```python
from build123d import *

# Parameters (mm, degrees)
F0_W     = 55
F0_H     = 55
F1_DEPTH = 20
F3_W     = 28
F3_H     = 28
F4_DEPTH = 13
F5_W     = 55
F5_H     = 55
F5_W_2   = 43
F5_H_2   = 43
F6_DEPTH = 9
F8_DEPTH = 22.5


with BuildPart() as f1:
    # F0 (on Top) → F1 (new body)
    with BuildSketch(Plane.XY):
        Rectangle(F0_W, F0_H)
    extrude(amount=F1_DEPTH)

    # F3 (on face) → F4 (cut, through all)
    with BuildSketch(Plane.XY.offset(20)):
        Rectangle(F3_W, F3_H)
    extrude(amount=-F4_DEPTH, mode=Mode.SUBTRACT)

    # F5 (on face) → F6 (cut)
    with BuildSketch(Plane.XY.offset(20)):
        Rectangle(F5_W, F5_H)
        Rectangle(F5_W_2, F5_H_2, mode=Mode.SUBTRACT)
    extrude(amount=-F6_DEPTH, mode=Mode.SUBTRACT)

    # F7 (on Front) → F8 (cut, symmetric)
    with BuildSketch(Plane.XZ):
        Polygon((21.5, 11), (21.5, 18), (17.5, 11), align=None)
    extrude(amount=F8_DEPTH, both=True, mode=Mode.SUBTRACT)


solid = f1.part
```
Source: CAD feature listing. Evaluate the final solid. Frame: model axes, mm. A direction names the side the tool comes from. Coordinates: 2 decimals unless noted, no trailing zeros. Loops run counter-clockwise (first coordinate to the right, second up) from the corner with the lowest first, then second, coordinate; pieces in that order, holes last. Notation, with made-up numbers: (-13, 81) -> (17, 81) arc R20 ccw to (17, 92) -> close; hole circle Ø8 at (10, -7). An arc over 180 degrees is marked (long way). One line per item, written item: value. Start each with the question number.
Q1. Contact query for flat-ended pins moving along their axis: P1, Ø1.6, axis at y = -2, z = 19, coming from the +X side; P2, Ø4, axis at x = 4, y = -7, coming from the +Z side; P3, Ø4.5, axis at y = 2, z = 15, coming from the -X side. Output: stop coordinate, or through.
Q2. Mould query, pull axis X, two halves, no side actions, for faces 1 (the face through (21.5, 0, 19)), 2 (the face through (-14, 0, 14)), 3 (the face through (18, 0, 11)). Classes: pulls with the +X half, pulls with the -X half, needs draft (parallel to the pull), parting line crosses it, or undercut.
Q3. Section query A-A, the plane x = 19.5. Return the cut outline in (y, z), and give its area (4 significant figures).
Q4. Section query B-B, the plane z = 7.75. Return the cut outline in (x, y), and give its area (3 significant figures).
Q5. Section query C-C, the plane y = -15. Return the cut outline in (x, z), and give its area (3 significant figures).
Q6. Line query: line 1 along Y through (x, z) = (12, 13.25); line 2 along X through (y, z) = (1, 9.75). Output: solid intervals per line, ascending.
Q7. Set-up query: faces 4 (the face through (0, 21.5, 16)), 5 (the face through (0, -14, 14)), 6 (the face through (0, -21.5, 16)), 7 (the face through (-21.5, 0, 16)), 8 (the face through (19.5, -0.3, 14.5)). Return all of +Z, -Z, +X, -X, +Y, -Y with unobstructed straight access to the full face (end or side cutting, diameter ignored); none if empty.
Q8. Section query D-D, the plane x = 0. Return the cut outline in (y, z).
Results:
1. P1: x = 21.5
1. P2: z = 7
1. P3: x = -21.5
2. face 1: pulls with the +X half
2. face 2: undercut
2. face 3: needs draft
3. outline: (-27.5, 0) -> (27.5, 0) -> (27.5, 11) -> (-27.5, 11) -> close; (-21.5, 14.5) -> (21.5, 14.5) -> (21.5, 20) -> (-21.5, 20) -> close
3. area: 841.5 mm^2
4. outline: (-27.5, -27.5) -> (27.5, -27.5) -> (27.5, 27.5) -> (-27.5, 27.5) -> close; hole (-14, -14) -> (14, -14) -> (14, 14) -> (-14, 14) -> close
4. area: 2,240 mm^2
5. outline: (-27.5, 0) -> (27.5, 0) -> (27.5, 11) -> (17.5, 11) -> (21.5, 18) -> (21.5, 20) -> (-21.5, 20) -> (-21.5, 11) -> (-27.5, 11) -> close
5. area: 978 mm^2
6. line 1: -21.5 to -14, 14 to 21.5
6. line 2: -27.5 to -14, 14 to 27.5
7. face 4: +Z, +X, -X, +Y
7. face 5: +Z
7. face 6: +Z, +X, -X, -Y
7. face 7: +Z, -X, +Y, -Y
7. face 8: +X, +Y, -Y
8. outline: (-27.5, 0) -> (27.5, 0) -> (27.5, 11) -> (21.5, 11) -> (21.5, 20) -> (14, 20) -> (14, 7) -> (-14, 7) -> (-14, 20) -> (-21.5, 20) -> (-21.5, 11) -> (-27.5, 11) -> close
